Could you check a few things on this model? Use its own coordinates, in mm. Round coordinates to 2 decimals unless told otherwise and drop trailing zeros. Order: outer loops, then holes, each group sorted by start corner. A loop starts at its lowest first (then second) coordinate and runs counter-clockwise, first axis right, second up. Notation, with made-up numbers: (13.5, 16) - (25.5, 16) arc R11 cw to (25.5, 24) - close; hole circle Ø2 at (25.5, -6.75). An arc over 180 degrees is marked (long way). Return JSON: item names as keys, results as strings. Group by question number.
from build123d import *

# Parameters (mm, degrees)
F1_DEPTH      = 12.7
F2_DEPTH      = 38.1
F3_DEPTH      = 25.4
F3_DEPTH_BACK = 12.7


with BuildPart() as f1:
    # F0 (on Right) → F1 (new body)
    with BuildSketch(Plane.YZ):
        with BuildLine():
            ThreePointArc((12.7, 25.4), (0, 38.1), (-12.7, 25.4))
            Line((-12.7, 25.4), (-12.7, 0))
            ThreePointArc((-12.7, 0), (0, -12.7), (12.7, 0))
            Line((12.7, 0), (12.7, 25.4))
        make_face()
        with BuildLine():
            ThreePointArc((0, 6.35), (4.4901280605, 4.4901280605), (6.35, 0))
            ThreePointArc((6.35, 0), (-4.4901280605, -4.4901280605), (0, 6.35))
        make_face(mode=Mode.SUBTRACT)
        with BuildLine():
            ThreePointArc((6.35, 25.4), (4.4901280605, 20.9098719395), (0, 19.05))
            ThreePointArc((0, 19.05), (-4.4901280605, 29.8901280605), (6.35, 25.4))
        make_face(mode=Mode.SUBTRACT)
    extrude(amount=F1_DEPTH)

    # F0 (on Right) → F2 (join)
    with BuildSketch(Plane.YZ):
        with BuildLine():
            ThreePointArc((0, 6.35), (-4.4901280605, -4.4901280605), (6.35, 0))
            ThreePointArc((6.35, 0), (4.4901280605, 4.4901280605), (0, 6.35))
        make_face()
    extrude(amount=F2_DEPTH)

    # F0 (on Right) → F3 (join, two sides)
    with BuildSketch(Plane.YZ) as f3_sk:
        with BuildLine():
            ThreePointArc((6.35, 25.4), (-4.4901280605, 29.8901280605), (0, 19.05))
            ThreePointArc((0, 19.05), (4.4901280605, 20.9098719395), (6.35, 25.4))
        make_face()
    extrude(amount=-F3_DEPTH)
    extrude(f3_sk.sketch, amount=F3_DEPTH_BACK)


solid = f1.part
1) If I drill on line 1 along X through (y, z) = (-10.25, 7); line 2 along Y through (x, z) = (-15.5, 25.5); line 3 along X through (y, z) = (-2.5, 28), over which ranges is the centre line in solid material (lowest first)? Write a range as from..to.
2) I want a section at C-C, the plane z = 3.5. List the corners of the cut face in (x, y) for me.
3) Will these pins go through, and if not, where does the flat tip stop? pin 1 (4 mm diameter, centred on x = -12, y = 1, fed in from -Z); pin 2 (3 mm diameter, centred on x = 9, y = -4, fed in from -Z); pin 3 (1 mm diameter, centred on x = 14.5, y = -4, fed in from +Z); pin 4 (1.5 mm diameter, centred on x = 14, z = 30.5, fed in from -Y).
4) I want a section at B-B, the plane x = 30. List the corners of the cut face in (y, z) for me.
5) I want a section at D-D, the plane x = 9.5. List the corners of the cut face in (y, z) for me.
6) I want a section at A-A, the plane y = 3. List the corners of the cut face in (x, z) for me, plus the area to 3 significant figures.
Outcome:
{
 "1": {"line 1": "0..12.7", "line 2": "-6.35..6.35", "line 3": "-25.4..12.7"},
 "2": {"outline": "(0, -12.7) - (12.7, -12.7) - (12.7, -5.3) - (38.1, -5.3) - (38.1, 5.3) - (12.7, 5.3) - (12.7, 12.7) - (0, 12.7) - close"},
 "3": {"pin 1": "z = 19.05", "pin 2": "z = -12.45", "pin 3": "z = 5.3", "pin 4": "through"},
 "4": {"outline": "circle Ø12.7 at (0, 0)"},
 "5": {"outline": "(-12.7, 0) arc R12.7 ccw to (12.7, 0) - (12.7, 25.4) arc R12.7 ccw to (-12.7, 25.4) - close"},
 "6": {"outline": "(-25.4, 19.8) - (0, 19.8) - (0, -12.34) - (12.7, -12.34) - (12.7, -5.6) - (38.1, -5.6) - (38.1, 5.6) - (12.7, 5.6) - (12.7, 37.74) - (0, 37.74) - (0, 31) - (-25.4, 31) - close", "area": "1,200 mm^2"}
}
